Can you work these out from the drawing? Everything is in mm from the part's minimum corner. Round coordinates to 2 decimals unless told otherwise and drop trailing zeros. Loops run counter-clockwise (first coordinate to the right, second up) from the corner with the lowest first, then second, coordinate; pieces in that order, holes last. Notation, with made-up numbers: (69, -31.75) -> (127, -31.75) arc R17 ccw to (127, -4.75) -> close; hole circle Ø4 at (40.25, -2.75). An arc over 180 degrees is marked (long way). Answer as a JSON object with one key per item and string values.
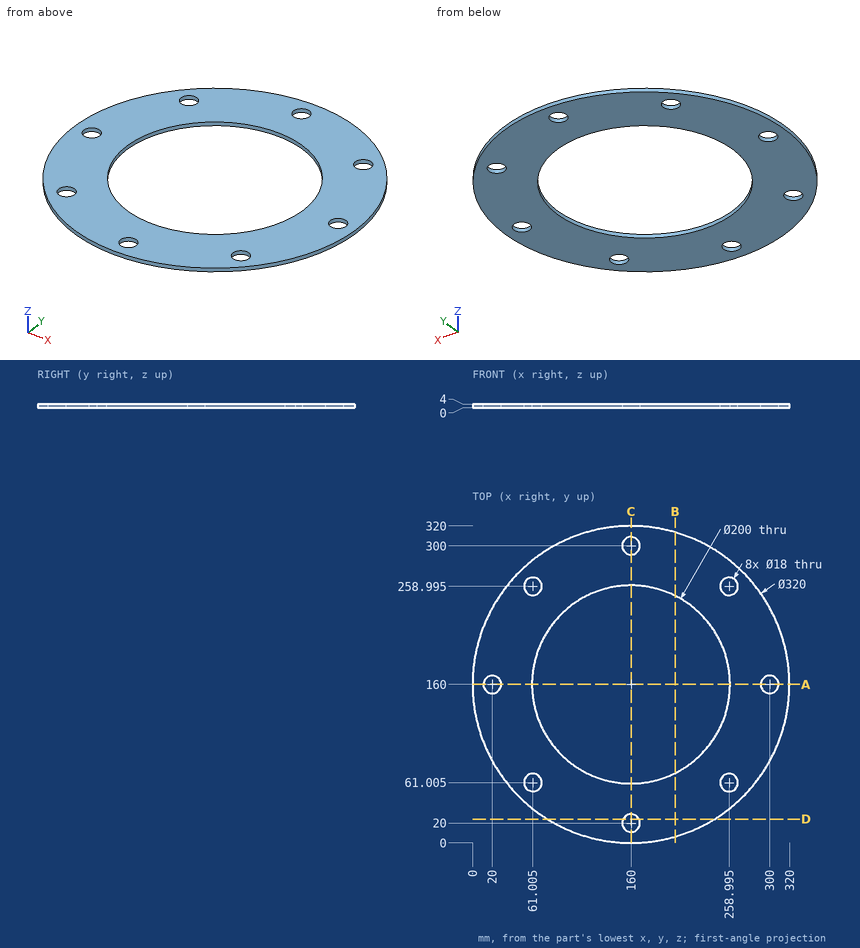
Q1. I'm going to push flat-ended pins straight in: pin 1 (1 mm diameter, centred on y = 247, z = 1, fed in from -X); pin 2 (2 mm diameter, centred on x = 110, z = 2.5, fed in from +Y); pin 3 (2 mm diameter, centred on x = 271.5, z = 3, fed in from +Y); pin 4 (14.5 mm diameter, centred on x = 258.99, y = 61.01, fed in from +Z) (3 decimals). Where does each tip first touch, or does it pass through?
Determined:
{"pin 1": "x = 25.4", "pin 2": "y = 312.31", "pin 3": "y = 275.71", "pin 4": "through"}
Q2. I want a section at D-D, the plane y = 24. Write out the boundary of the cut face in (x, z), then the cut area to 3 significant figures.
Determined:
{"outline": "(75.71, 0) -> (151.94, 0) -> (151.94, 4) -> (75.71, 4) -> close; (168.06, 0) -> (244.29, 0) -> (244.29, 4) -> (168.06, 4) -> close", "area": "610 mm²"}
Q3. I want a section at B-B, the plane x = 204.5. Write out the boundary of the cut face in (y, z).
Determined:
{"outline": "(6.31, 0) -> (70.45, 0) -> (70.45, 4) -> (6.31, 4) -> close; (249.55, 0) -> (313.69, 0) -> (313.69, 4) -> (249.55, 4) -> close"}
Q4. I want a section at A-A, the plane y = 160. Write out the boundary of the cut face in (x, z), then the cut area to 3 significant figures.
Determined:
{"outline": "(0, 0) -> (11, 0) -> (11, 4) -> (0, 4) -> close; (29, 0) -> (60, 0) -> (60, 4) -> (29, 4) -> close; (260, 0) -> (291, 0) -> (291, 4) -> (260, 4) -> close; (309, 0) -> (320, 0) -> (320, 4) -> (309, 4) -> close", "area": "336 mm²"}
Q5. If I drill on L1, parallel to Y at x = 160, z = 1.3; L2, parallel to X at y = 251.5, z = 1.65 (1 decimal); L3, parallel to Y at x = 20.5, z = 0.85, over which ranges is the centre line in solid material (lowest first)? Write a range as [from, to].
Determined:
{"L1": "[0, 11], [29, 60], [260, 291], [309, 320]", "L2": "[28.7, 56], [66, 119.7], [200.3, 254], [264, 291.3]", "L3": "[81.64, 151.01], [168.99, 238.36]"}
